Autodesk Inventor part; units mm, degrees
ref_plane "YZ Plane" through (0, 0, 0) normal (1, 0, 0) x (0, 1, 0)
ref_plane "XZ Plane" through (0, 0, 0) normal (0, 1, 0) x (-1, 0, 0)
ref_plane "XY Plane" through (0, 0, 0) normal (0, 0, 1) x (1, 0, 0)
sketch "Sketch1" plane through (0, 0, 0) normal (1, 0, 0) x (0, 1, 0)
  line L0 (0, 0) -> (-18, 0)
  line L1 (-18, 0) -> (-18, -22)
  line L2 (-18, -22) -> (0, -22)
  line L3 (0, -22) -> (0, 0)
  dimension "d0" = 18
  dimension "d1" = 22
extrude "Extrusion1" add sketch "Sketch1" along normal blind 4
chamfer "Chamfer1" distance 0.3 angle 45 12 edges at (4, 0, -11) (0, 0, -11) (2, 0, -22) (4, -9, 0) (2, 0, 0) (0, -9, -22) (2, -18, -22) (4, -9, -22) (4, -18, -11) (0, -18, -11) (0, -9, 0) (2, -18, 0)
sketch "Sketch2" plane through (0.3, -17.7, 0) normal (0, 0, 1) x (1, 0, 0)
  line L0 (-0.3, 17.4) -> (-0.3, 0)
  line L1 (3.4, 17.7) -> (0, 17.7)
  line L2 (0, -0.3) -> (3.4, -0.3)
  point P0 (-0.3, 17.7)
  point P1 (1.7, 14.7)
  point P2 (1.7, 2.7)
  dimension "d7" = 2
  dimension "d8" = 2
  dimension "d9" = 3
  dimension "d10" = 3
hole "Hole1" at (2, -3, 0) at (2, -15, 0) direction (0, 0, -1) diameter 1.567 depth 6.3 tip angle 118
sketch "Sketch3" plane through (3.7, -17.7, -22) normal (0, 0, -1) x (-1, 0, 0)
  circle A0 centre (1.7, 2.7) radius 0.7835
  circle A1 centre (1.7, 14.7) radius 0.7835
  point P0 (3.7, 17.7)
  point P1 (1.7, 2.7)
  point P2 (1.7, 14.7)
hole "Hole2" at (2, -15, -22) at (2, -3, -22) direction (0, 0, 1) diameter 1.567 depth 6.3 tip angle 118
sketch "Sketch4" plane through (0, 0, 0) normal (-1, 0, 0) x (0, 0, 1)
  line L0 (-22, -0.3) -> (-22, -17.7)
  line L1 (-0.3, 0) -> (-21.7, 0)
  point P0 (0, 0)
  point P1 (-11, -9)
  dimension "d25" = 11
  dimension "d26" = 9
hole "Hole3" at (0, -9, -11) direction (1, 0, 0) diameter 4 depth 6.3 tip angle 118
properties part number "Ramka4" material "Steel(1)"
The model under review builds one solid part; all positions refer to its coordinate system, in mm. A direction names the side the tool comes from. Give positions to 0.01 mm unless a question says otherwise; leave off trailing zeros. Write each loop counter-clockwise with the first axis right and the second up, starting at its lowest first coordinate (ties: lowest second). Pieces come first, ordered by that corner, then holes. Notation, with made-up numbers: (-22.75, 53.5) -> (20.25, 53.5) arc R19 cw to (20.25, 59.5) -> close; hole circle Ø4 at (64.25, 5.25). An arc over 180 degrees is marked (long way). Answer in a Markdown table with one row per item.
1) Tool access review of faces 4 (the cylindrical face through (2.765, -14.83, -3.194)), 5 (the flat face through (2, -18, -11)), 6 (the cylindrical face through (2.695, -2.638, -18.806)): name each direction out of +Z, -Z, +X, -X, +Y, -Y from which nothing blocks a thin tool from reaching the whole face with its end or side.
Worked answers:
| item | result |
|---|---|
| face 4 | +Z |
| face 5 | +Z, -Z, +X, -X, -Y |
| face 6 | -Z |
2) Clearance check with flat-ended pins moving along their axes: P1, Ø1.4, axis at x = 2, y = -15, coming from the +Z side; P2, Ø3.5, axis at y = -9, z = -11, coming from the -X side. State where each tip first meets the part, or that it passes through.
Worked answers:
| item | result |
|---|---|
| P1 | z = -6.35 |
| P2 | through |
3) Add section A-A on y = -9. State the section outline as (x, z) points, plus the area to 3 significant figures.
Worked answers:
| item | result |
|---|---|
| outline | (0, -21.7) -> (0.3, -22) -> (3.7, -22) -> (4, -21.7) -> (4, -13) -> (0, -13) -> close; (0, -9) -> (4, -9) -> (4, -0.3) -> (3.7, 0) -> (0.3, 0) -> (0, -0.3) -> close |
| area | 71.8 mm² |
4) For L1, parallel to X at y = -15, z = -17; L2, parallel to Y at x = 2, z = -2.75; L3, parallel to Y at x = 1.4, z = -4.75, list the stretches that pass through material, from the lowest coordinate up. Write a range as [from, to].
Worked answers:
| item | result |
|---|---|
| L1 | [0, 1.22], [2.78, 4] |
| L2 | [-18, -15.78], [-14.22, -3.78], [-2.22, 0] |
| L3 | [-18, -15.5], [-14.5, -3.5], [-2.5, 0] |
5) Add section C-C on z = -6. State the section outline as (x, y) points, plus the area to 3 significant figures.
Worked answers:
| item | result |
|---|---|
| outline | (0, -17.7) -> (0.3, -18) -> (3.7, -18) -> (4, -17.7) -> (4, -0.3) -> (3.7, 0) -> (0.3, 0) -> (0, -0.3) -> close; hole circle Ø1.57 at (2, -15); hole circle Ø1.57 at (2, -3) |
| area | 68.0 mm² |
6) Add section B-B on z = -11. State the section outline as (x, y) points.
Worked answers:
| item | result |
|---|---|
| outline | (0, -17.7) -> (0.3, -18) -> (3.7, -18) -> (4, -17.7) -> (4, -11) -> (0, -11) -> close; (0, -7) -> (4, -7) -> (4, -0.3) -> (3.7, 0) -> (0.3, 0) -> (0, -0.3) -> close |
7) Mouldability with a two-part tool opening along Y and no side actions: class faces 1 (the flat face through (2, 0, -11)), 2 (the flat face through (2, -9, 0)), 3 (the conical face through (2.006, -15.136, -15.311)) as +Y half, -Y half, draft (parallel to the pull), parting line (faces both ways), or undercut.
Worked answers:
| item | result |
|---|---|
| face 1 | +Y half |
| face 2 | draft |
| face 3 | undercut |
